Solid Edge part; units mm, degrees
sketch "Sketch1" plane through (0, 0, 0) normal (0, -1, 0) x (1, 0, 0)
  line L0 (-39.6277, 18) -> (56.9723, 18)
  line L1 (56.9723, 18) -> (56.9723, 24)
  line L2 (56.9723, 24) -> (-39.6277, 24)
  line L3 (-39.6277, 24) -> (-39.6277, 18)
  dimension "D1" = 56.9723
  dimension "D2" = 39.6277
extrude "Protrusion1" add sketch "Sketch1" against normal blind 95
sketch "Sketch2" plane through (8.6723, 47.5, 24) normal (0, 0, 1) x (-1, 0, 0)
  circle A0 centre (-40.48, 36.4) radius 5
  circle A1 centre (-40.48, 5) radius 5
  circle A2 centre (-40.48, -30.8) radius 5
  circle A3 centre (42.5, -30.8) radius 5
  circle A4 centre (42.5, 4.8905) radius 5
  circle A5 centre (42.5, 36.4) radius 5
extrude "ExtrudedCutout_1" cut sketch "Sketch2" against normal blind 37.274
sketch "Sketch3" plane through (8.6723, 47.5, 24) normal (0, 0, 1) x (-1, 0, 0)
  circle A0 centre (-8.5, 29.5904) radius 2.2
  circle A1 centre (14, 16.6) radius 2.2
  circle A2 centre (-8.5, 3.6096) radius 2.2
  circle A3 centre (2, -10.4) radius 2.2
  circle A4 centre (24.5, 2.5904) radius 2.2
  circle A5 centre (24.5, -23.3904) radius 2.2
extrude "ExtrudedCutout_2" cut sketch "Sketch3" against normal blind 69.9248
sketch "Sketch4" plane through (8.6723, 47.5, 24) normal (0, 0, 1) x (-1, 0, 0)
  circle A0 centre (-1, 16.6) radius 10
  circle A1 centre (17, -10.4) radius 10
extrude "ExtrudedCutout_3" cut sketch "Sketch4" against normal blind 48.6044
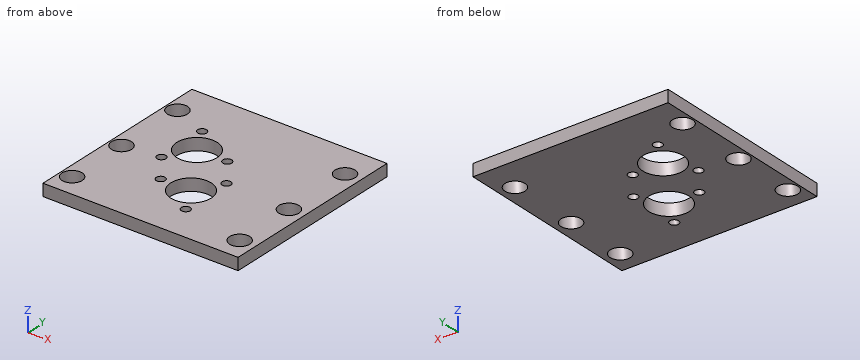
Check sheet for the modelled part. Datum: model origin and axes. Units: mm. Give positions to 0.01 mm unless a question says otherwise; leave off trailing zeros. Write each loop counter-clockwise with the first axis right and the second up, starting at its lowest first coordinate (ties: lowest second). Pieces come first, ordered by that corner, then holes. Notation, with made-up numbers: M 33,15.5 L 75,15.5 A17 cw 75,25.5 Z; hole C 2.25,23 d11. An arc over 180 degrees is marked long. Use one line per item in the form item = value.
(1) Material ranges on line 1 along X through (y, z) = (57.9, 21.25); line 2 along X through (y, z) = (30.9, 21.55); line 3 along Y through (x, z) = (-16.5, 22.1), recorded low to high.
Answer block:
line_1 = -39.63 to -18.33, 1.67 to 4.47, 8.87 to 56.97
line_2 = -39.63 to -7.53, -3.13 to -0.33, 19.67 to 56.97
line_3 = 0 to 42.81, 47 to 52.14, 63.66 to 68.8, 72.99 to 95
(2) Section check A-A on y = 11.1. Record the boundary of the cut face in (x, z), plus the area to 3 significant figures.
Answer block:
outline = M -39.63,18 L -38.83,18 L -38.83,24 L -39.63,24 Z; M -28.83,18 L 44.15,18 L 44.15,24 L -28.83,24 Z; M 54.15,18 L 56.97,18 L 56.97,24 L 54.15,24 Z
area = 460 mm2
(3) Section check B-B on x = 18. Record the boundary of the cut face in (y, z), plus the area to 3 significant figures.
Answer block:
outline = M 0,18 L 15.87,18 L 15.87,24 L 0,24 Z; M 19.95,18 L 25.36,18 L 25.36,24 L 19.95,24 Z; M 36.44,18 L 41.85,18 L 41.85,24 L 36.44,24 Z; M 45.93,18 L 95,18 L 95,24 L 45.93,24 Z
area = 455 mm2
(4) Section check C-C on z = 20.55. State how many separate pieces and enclosed holes the cut face has, plus the area to 3 significant figures.
Answer block:
separate_pieces = 1
enclosed_holes = 14
area = 7,990 mm2
(5) Section check D-D on y = 30.9. Record the boundary of the cut face in (x, z), plus the area to 3 significant figures.
Answer block:
outline = M -39.63,18 L -7.53,18 L -7.53,24 L -39.63,24 Z; M -3.13,18 L -0.33,18 L -0.33,24 L -3.13,24 Z; M 19.67,18 L 56.97,18 L 56.97,24 L 19.67,24 Z
area = 433 mm2
(6) Depth check by flat-ended pin: P1, Ø6, axis at x = -33.83, y = 42.61, coming from the -Z side. Enter the tip coordinate at first touch or a pass-through.
Answer block:
P1 = through
